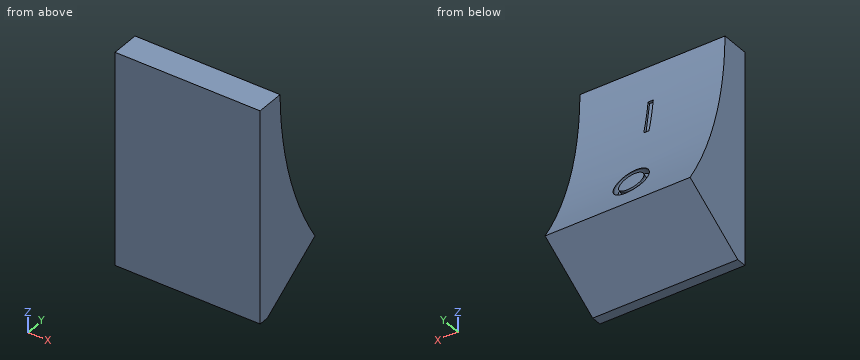
Autodesk Inventor part; units mm, degrees
ref_plane "to_body_XY" through (0, 0, 0) normal (0, 1, 0) x (1, 0, 0)
ref_plane "to_body_YZ" through (0, 0, 0) normal (1, 0, 0) x (0, 0, -1)
ref_plane "to_body_ZX" through (0, 0, 0) normal (0, 0, -1) x (0, 1, 0)
sketch "Sketch_2" plane through (0, 0, 0) normal (1, 0, 0) x (0, 1, 0)
  line L0 (2.0701, 7.7724) -> (0, 7.7724)
  line L1 (0, 7.7724) -> (0, -7.7724)
  line L2 (0, -7.7724) -> (0.7455, -7.7724)
  line L3 (0.7455, -7.7724) -> (5.6896, -4.6127)
  arc A0 (2.0701, 7.7724) -> (5.6896, -4.6127) centre (25.9234, 8.0219) ccw
extrude "Extrusion1" add sketch "Sketch_2" along normal mid plane 10.5918
sketch "Sketch_3" plane through (0, 3.2333, 0.3287) normal (0, 0.9239, 0.3827) x (1, 0, 0)
  circle A0 centre (0, 2.54) radius 1.27
  circle A1 centre (0, 2.54) radius 0.889
extrude "Extrusion2" cut sketch "Sketch_3" along normal mid plane 0.762
sketch "Sketch_4" plane through (0, 3.2333, 0.3287) normal (0, 0.9877, 0.1564) x (1, 0, 0)
  line L0 (-0.1905, -4.826) -> (0.1905, -4.826)
  line L1 (0.1905, -4.826) -> (0.1905, -2.286)
  line L2 (0.1905, -2.286) -> (-0.1905, -2.286)
  line L3 (-0.1905, -2.286) -> (-0.1905, -4.826)
extrude "Extrusion3" cut sketch "Sketch_4" along normal mid plane 0.762
ref_plane "to_body_XY" through (0, 0, 0) normal (0, 1, 0) x (1, 0, 0)
ref_plane "to_body_YZ" through (0, 0, 0) normal (1, 0, 0) x (0, 0, -1)
ref_plane "to_body_ZX" through (0, 0, 0) normal (0, 0, -1) x (0, 1, 0)
properties part number "CWSB2-nonillumin_rocker"
Here's how the part is built. I have some questions about the finished solid (model axes, mm). Give positions to 0.01 mm unless a question says otherwise; leave off trailing zeros. Loops run counter-clockwise (first coordinate to the right, second up) from the corner with the lowest first, then second, coordinate; pieces in that order, holes last. Notation, with made-up numbers: (83.5, 49) -> (109.5, 49) arc R26 ccw to (109.5, 76) -> close; hole circle Ø7 at (80.5, -26.75). An arc over 180 degrees is marked (long way). Answer as a JSON object with one key per item and string values. Group by question number.
Item 1: Imagine slicing it at A-A on x = 4. Write out the boundary of the cut face in (y, z).
Item 2: I need wall thicknesses on L1, parallel to Y at x = -4, z = 6.75; L2, parallel to Y at x = -4, z = 0.5; L3, parallel to Z at x = -3.75, y = 5.15. Which ranges of each line are inside material? Lowest first, please.
Item 3: Will these pins go through, and if not, where does the flat tip stop? pin 1 (1.5 mm diameter, centred on x = -3.5, y = 3, fed in from -Z); pin 2 (1.5 mm diameter, centred on y = 4, z = 5.5, fed in from -X); pin 3 (3 mm diameter, centred on x = -1.5, z = 1, fed in from +Y).
Item 4: Imagine slicing it at B-B on y = 1.45. Write out the boundary of the cut face in (x, z).
Item 5: Imagine slicing it at C-C on z = 2. Write out the boundary of the cut face in (x, y).
Answer list:
{
 "1": {"outline": "(0, -7.77) -> (0.75, -7.77) -> (5.69, -4.61) arc R23.85 cw to (2.07, 7.77) -> (0, 7.77) -> close"},
 "2": {"L1": "y = 0 to 2.1", "L2": "y = 0 to 3.29", "L3": "z = -4.96 to -3.7"},
 "3": {"pin 1": "stops at z = -6.81", "pin 2": "passes through", "pin 3": "stops at y = 3.64"},
 "4": {"outline": "(-5.3, -7.32) -> (5.3, -7.32) -> (5.3, 7.77) -> (-5.3, 7.77) -> close"},
 "5": {"outline": "(-5.3, 0) -> (5.3, 0) -> (5.3, 2.84) -> (-5.3, 2.84) -> close"}
}
